from build123d import *

# Parameters (mm, degrees)
SKETCH1_R             = 27
SKETCH1_R_2           = 1.25
SKETCH1_R_3           = 20
BOSS_EXTRUDE1_DEPTH   = 3
SKETCH1_R_4           = 9.5
SKETCH1_R_5           = 4
BOSS_EXTRUDE1_2_DEPTH = 3
BOSS_EXTRUDE2_DEPTH   = 3


with BuildPart() as part:
    # Sketch1 → Boss-Extrude1 (new body)
    with BuildSketch(Plane.XY):
        Circle(SKETCH1_R)
        with Locations((23.5, 0)):
            Circle(SKETCH1_R_2, mode=Mode.SUBTRACT)
        with Locations((0, -23.5)):
            Circle(SKETCH1_R_2, mode=Mode.SUBTRACT)
        with Locations((-23.5, 0)):
            Circle(SKETCH1_R_2, mode=Mode.SUBTRACT)
        with Locations((0, 23.5)):
            Circle(SKETCH1_R_2, mode=Mode.SUBTRACT)
        Circle(SKETCH1_R_3, mode=Mode.SUBTRACT)
    extrude(amount=BOSS_EXTRUDE1_DEPTH)



with BuildPart() as body_2:
    # Sketch1 → Boss-Extrude1 2 (new body)
    with BuildSketch(Plane.XY):
        Circle(SKETCH1_R_4)
        with Locations((6.75, 0)):
            Circle(SKETCH1_R_2, mode=Mode.SUBTRACT)
        with Locations((0, -6.75)):
            Circle(SKETCH1_R_2, mode=Mode.SUBTRACT)
        with Locations((-6.75, 0)):
            Circle(SKETCH1_R_2, mode=Mode.SUBTRACT)
        with Locations((0, 6.75)):
            Circle(SKETCH1_R_2, mode=Mode.SUBTRACT)
        Circle(SKETCH1_R_5, mode=Mode.SUBTRACT)
    extrude(amount=BOSS_EXTRUDE1_2_DEPTH)


with BuildPart() as part_1:
    add(part.part)

    add(body_2.part)  # Boss-Extrude2 merges body 2
    # Sketch2 → Boss-Extrude2 (add)
    with BuildSketch(Plane.XY):
        with BuildLine():
            ThreePointArc((-13.918195932, 1.194775158), (-11.982498043, 1.275378496), (-10.222750069, 2.085755129))
            Line((-10.222750069, 2.085755129), (-9.030872227, 2.948448204))
            Line((-9.030872227, 2.948448204), (-9.030872227, -2.948448204))
            Line((-9.030872227, -2.948448204), (-10.222750069, -2.085755129))
            ThreePointArc((-10.222750069, -2.085755129), (-11.982498043, -1.275378496), (-13.918195932, -1.194775158))
            Line((-13.918195932, -1.194775158), (-19.887594178, -2.117450782))
            Line((-19.887594178, -2.117450782), (-20.214883486, 0))
            Line((-20.214883486, 0), (-19.887594178, 2.117450782))
            Line((-19.887594178, 2.117450782), (-13.918195932, 1.194775158))
        make_face()
        with BuildLine():
            Line((0, 20.214883486), (2.117450782, 19.887594178))
            Line((2.117450782, 19.887594178), (1.194775158, 13.918195932))
            ThreePointArc((1.194775158, 13.918195932), (1.275378496, 11.982498043), (2.085755129, 10.222750069))
            Line((2.085755129, 10.222750069), (2.948448204, 9.030872227))
            Line((2.948448204, 9.030872227), (-2.948448204, 9.030872227))
            Line((-2.948448204, 9.030872227), (-2.085755129, 10.222750069))
            ThreePointArc((-2.085755129, 10.222750069), (-1.275378496, 11.982498043), (-1.194775158, 13.918195932))
            Line((-1.194775158, 13.918195932), (-2.117450782, 19.887594178))
            Line((-2.117450782, 19.887594178), (0, 20.214883486))
        make_face()
        with BuildLine():
            Line((19.887594178, -2.117450782), (13.918195932, -1.194775158))
            ThreePointArc((13.918195932, -1.194775158), (11.982498043, -1.275378496), (10.222750069, -2.085755129))
            Line((10.222750069, -2.085755129), (9.030872227, -2.948448204))
            Line((9.030872227, -2.948448204), (9.030872227, 2.948448204))
            Line((9.030872227, 2.948448204), (10.222750069, 2.085755129))
            ThreePointArc((10.222750069, 2.085755129), (11.982498043, 1.275378496), (13.918195932, 1.194775158))
            Line((13.918195932, 1.194775158), (19.887594178, 2.117450782))
            Line((19.887594178, 2.117450782), (20.214883486, 0))
            Line((20.214883486, 0), (19.887594178, -2.117450782))
        make_face()
        with BuildLine():
            Line((2.117450782, -19.887594178), (1.194775158, -13.918195932))
            ThreePointArc((1.194775158, -13.918195932), (1.275378496, -11.982498043), (2.085755129, -10.222750069))
            Line((2.085755129, -10.222750069), (2.948448204, -9.030872227))
            Line((2.948448204, -9.030872227), (-2.948448204, -9.030872227))
            Line((-2.948448204, -9.030872227), (-2.085755129, -10.222750069))
            ThreePointArc((-2.085755129, -10.222750069), (-1.275378496, -11.982498043), (-1.194775158, -13.918195932))
            Line((-1.194775158, -13.918195932), (-2.117450782, -19.887594178))
            Line((-2.117450782, -19.887594178), (0, -20.214883486))
            Line((0, -20.214883486), (2.117450782, -19.887594178))
        make_face()
    extrude(amount=BOSS_EXTRUDE2_DEPTH)


solid = part_1.part
Could you check a few things on this model? Use its own coordinates, in mm. Give positions to 0.01 mm unless a question says otherwise; leave off trailing zeros. Loops run counter-clockwise (first coordinate to the right, second up) from the corner with the lowest first, then second, coordinate; pieces in that order, holes last. Notation, with made-up numbers: (-35.5, -24.75) -> (20.5, -24.75) arc R37 ccw to (20.5, 14.25) -> close; hole circle Ø5 at (23.5, -21). An arc over 180 degrees is marked (long way). Return JSON: item names as keys, results as strings.
Item 1: I'm going to push flat-ended pins straight in: pin 1 (1.5 mm diameter, centred on x = 0, y = 23.5, fed in from +Z); pin 2 (3 mm diameter, centred on x = -6.75, y = 0, fed in from +Z). Where does each tip first touch, or does it pass through?
Geometry results:
{"pin 1": "passes through", "pin 2": "stops at z = 3"}
Item 2: We'd pull the mould along Y, two halves only. Please class faces 1 (the cylindrical face through (1.27, -12.01, 1.48)), 2 (the cylindrical face through (-5.85, -26.36, 1.48)): +Y half, -Y half, draft (parallel to the pull), parting line (faces both ways), or undercut.
Geometry results:
{"face 1": "undercut", "face 2": "parting line"}
Item 3: If we section it at A-A on y = 23.5: List the corners of the cut face in (x, z) for me.
Geometry results:
{"outline": "(-13.29, 0) -> (-1.25, 0) -> (-1.25, 3) -> (-13.29, 3) -> close; (1.25, 0) -> (13.29, 0) -> (13.29, 3) -> (1.25, 3) -> close"}
Item 4: I need wall thicknesses on L1, parallel to Y at x = 0, z = 1.4; L2, parallel to Y at x = -7, z = 0.5 (3 decimals); L3, parallel to Y at x = -1, z = 0.2. Which ranges of each line are inside material? Lowest first, please. Write a range as from..to.
Geometry results:
{"L1": "y = -27..-24.75, -22.25..-8, -5.5..-4, 4..5.5, 8..22.25, 24.75..27", "L2": "y = -26.077..-18.735, -6.423..-1.225, 1.225..6.423, 18.735..26.077", "L3": "y = -26.98..-24.25, -22.75..-7.5, -6..-3.87, 3.87..6, 7.5..22.75, 24.25..26.98"}
Item 5: If we section it at B-B on x = 6.75: List the corners of the cut face in (y, z) for me, plus the area to 3 significant figures.
Geometry results:
{"outline": "(-26.14, 0) -> (-18.83, 0) -> (-18.83, 3) -> (-26.14, 3) -> close; (-6.68, 0) -> (-1.25, 0) -> (-1.25, 3) -> (-6.68, 3) -> close; (1.25, 0) -> (6.68, 0) -> (6.68, 3) -> (1.25, 3) -> close; (18.83, 0) -> (26.14, 0) -> (26.14, 3) -> (18.83, 3) -> close", "area": "76.5 mm²"}
Item 6: If we section it at D-D on z = 2.3: Count the separate pieces of the cut face and the enclosed holes in it, plus the area to 3 significant figures.
Geometry results:
{"separate pieces": "1", "enclosed holes": "13", "area": "1,370 mm²"}
